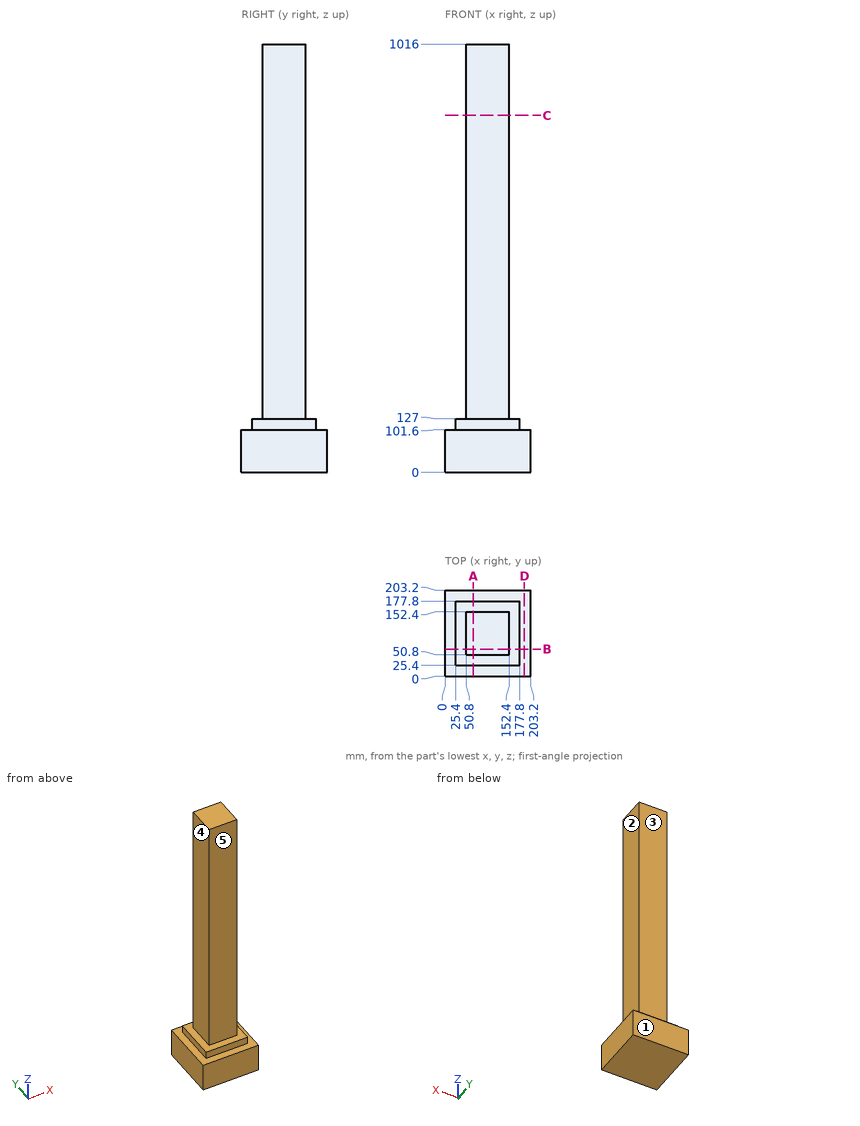
Could you check a few things on this drawing? It's one solid part, dimensions in mm from its lowest x, y, z. A direction names the side the tool comes from. Coordinates: 2 decimals unless noted, no trailing zeros. Loops run counter-clockwise (first coordinate to the right, second up) from the corner with the lowest first, then second, coordinate; pieces in that order, holes last.
1. We'd pull the mould along Y, two halves only. Please class the marked faces 3, 4 and 5: released by +Y, released by -Y, zero draft, split by the parting line, or undercut.
2. Imagine slicing it at D-D (x = 188). Please give me the cut outline in (y, z), and give its area (3 significant figures).
3. Imagine slicing it at C-C (z = 846.5). Please give me the cut outline in (x, y), and give its area (3 significant figures).
4. I need wall thicknesses on L1, parallel to Y at x = 104.5, z = 512.5; L2, parallel to Z at x = 156, y = 175. Which ranges of each line are inside material? Lowest first, please.
5. Imagine slicing it at A-A (x = 67). Please give me the cut outline in (y, z).
6. For P1, Ø4, axis at x = 138, z = 225, coming from the +Y side; P2, Ø4, axis at x = 29.5, y = 35.5, coming from the +Z side; P3, Ø12.5, axis at y = 97.5, z = 114, coming from the +X side, each with a flat end and sliding along its axis, tell me the tip position at first contact or that it passes through.
7. For the marked faces 1 and 2, which set-ups out of +Z, -Z, +X, -X, +Y, -Y let a thin tool reach every point of the face, with its end or its side?
Computed values:
1. face 3: released by +Y
1. face 4: zero draft
1. face 5: released by -Y
2. outline: (0, 0) - (203.2, 0) - (203.2, 101.6) - (0, 101.6) - close
2. area: 20,600 mm2
3. outline: (50.8, 50.8) - (152.4, 50.8) - (152.4, 152.4) - (50.8, 152.4) - close
3. area: 10,300 mm2
4. L1: y = 50.8 to 152.4
4. L2: z = 0 to 127
5. outline: (0, 0) - (203.2, 0) - (203.2, 101.6) - (177.8, 101.6) - (177.8, 127) - (152.4, 127) - (152.4, 1016) - (50.8, 1016) - (50.8, 127) - (25.4, 127) - (25.4, 101.6) - (0, 101.6) - close
6. P1: stops at y = 152.4
6. P2: stops at z = 127
6. P3: stops at x = 177.8
7. face 1: +Z, -Z, +X, -X, +Y
7. face 2: +Z, +X, +Y, -Y
